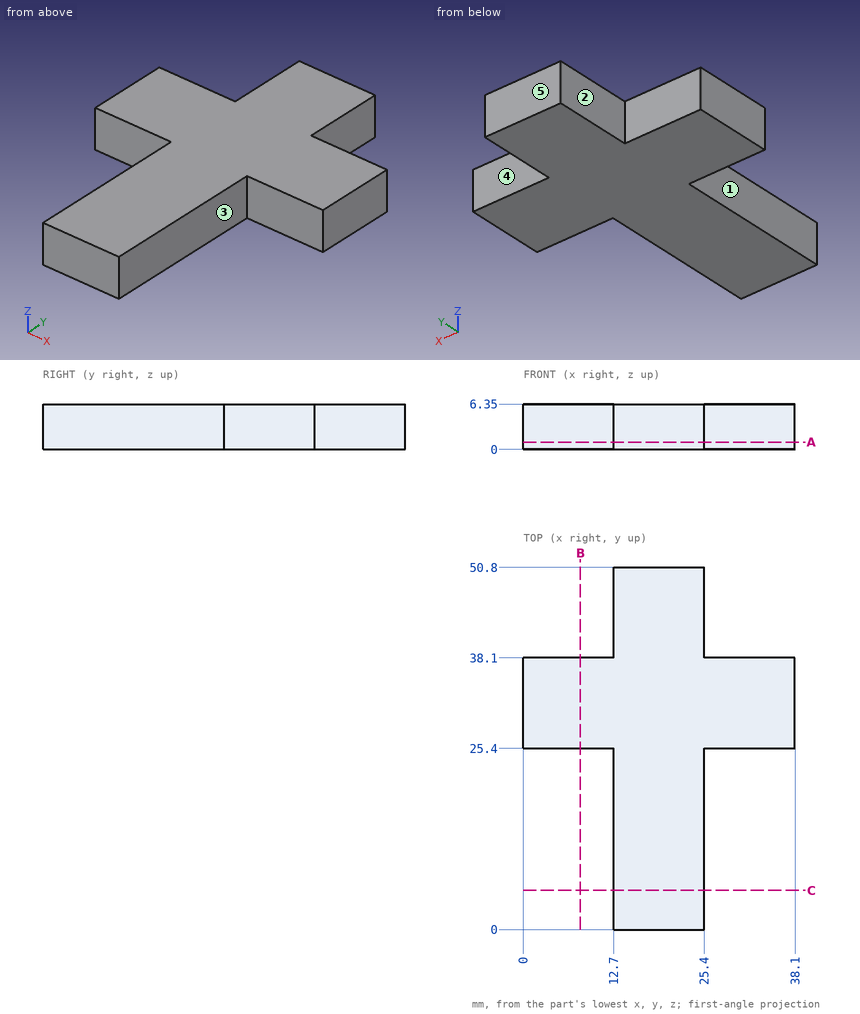
Can you work these out from the drawing? Everything is in mm from the part's minimum corner. A direction names the side the tool comes from. Give positions to 0.01 mm unless a question says otherwise; leave off trailing zeros. Order: outer loops, then holes, each group sorted by start corner. A loop starts at its lowest first (then second) coordinate and runs counter-clockwise, first axis right, second up.
Item 1: If we section it at B-B, the plane x = 8: Write out the boundary of the cut face in (y, z), plus the area to 3 significant figures.
Item 2: If we section it at C-C, the plane y = 5.5: Write out the boundary of the cut face in (x, z), plus the area to 3 significant figures.
Item 3: If we section it at A-A, the plane z = 1: Write out the boundary of the cut face in (x, y), plus the area to 3 significant figures.
Item 4: I need wall thicknesses on line 1 (X direction, y = 15, z = 6.25); line 2 (Y direction, x = 33, z = 3). Which ranges of each line are inside material? Lowest first, please.
Item 5: I'm going to push flat-ended pins straight in: pin 1 (1.9 mm diameter, centred on x = 5, z = 2.5, fed in from -Y); pin 2 (3 mm diameter, centred on y = 10, z = 2, fed in from +X); pin 3 (3 mm diameter, centred on y = 39.5, z = 5, fed in from +X). Where does each tip first touch, or does it pass through?
Item 6: For the marked faces 1, 2, 3, 4 and 5, which set-ups out of +Z, -Z, +X, -X, +Y, -Y let a thin tool reach every point of the face, with its end or its side?
Values:
1. outline: (25.4, 0) - (38.1, 0) - (38.1, 6.35) - (25.4, 6.35) - close
1. area: 80.6 mm2
2. outline: (12.7, 0) - (25.4, 0) - (25.4, 6.35) - (12.7, 6.35) - close
2. area: 80.6 mm2
3. outline: (0, 25.4) - (12.7, 25.4) - (12.7, 0) - (25.4, 0) - (25.4, 25.4) - (38.1, 25.4) - (38.1, 38.1) - (25.4, 38.1) - (25.4, 50.8) - (12.7, 50.8) - (12.7, 38.1) - (0, 38.1) - close
3. area: 968 mm2
4. line 1: x = 12.7 to 25.4
4. line 2: y = 25.4 to 38.1
5. pin 1: stops at y = 25.4
5. pin 2: stops at x = 25.4
5. pin 3: stops at x = 38.1
6. face 1: +Z, -Z, -X, -Y
6. face 2: +Z, -Z, -X, +Y
6. face 3: +Z, -Z, +X, -Y
6. face 4: +Z, -Z, +X, +Y
6. face 5: +Z, -Z, +X, -X, +Y
